from build123d import *

# Parameters (mm, degrees)
F0_W      = 76.2
F0_H      = 63.5
F1_DEPTH  = 50.8
F3_DEPTH  = 50.8
F4_W      = 19.05
F4_H      = 44.45
F5_DEPTH  = 38.1
F6_W      = 19.05
F6_H      = 19.05
F7_DEPTH  = 12.7
F10_DEPTH = 12.7
F11_R     = 3.175
F12_DEPTH = 69.851
F13_DEPTH = 31.75


with BuildPart() as f1:
    # F0 (on Front) → F1 (new body)
    with BuildSketch(Plane.XZ):
        with Locations((-7.4970987678, 21.3185883239)):
            Rectangle(F0_W, F0_H)
    extrude(amount=-F1_DEPTH)

    # F2 (on face) → F3 (cut)
    with BuildSketch(Plane.XZ):
        Polygon((-45.5970987678, 14.9685883239), (-45.5970987678, -10.4314116761), (-20.1970987678, -10.4314116761), align=None)
        Polygon((30.6029012322, 40.3685883239), (30.6029012322, 53.0685883239), (-7.4970987678, 53.0685883239), align=None)
    extrude(amount=-F3_DEPTH, mode=Mode.SUBTRACT)

    # F4 (on face) → F5 (join)
    with BuildSketch(Plane.YZ.offset(30.6029012322)):
        Polygon((19.05, 14.9685883239), (19.05, -10.4314116761), (50.8, -10.4314116761), (50.8, 14.9685883239), (38.1, 14.9685883239), align=None)
        with Locations((28.575, 37.1935883239)):
            Rectangle(F4_W, F4_H)
    extrude(amount=F5_DEPTH)

    # F6 (on face) → F7 (join)
    with BuildSketch(Plane(origin=(30.6029012322, 0, 0), x_dir=(0, -1, 0), z_dir=(-1, 0, 0))):
        with Locations((-28.575, 49.8935883239)):
            Rectangle(F6_W, F6_H)
    extrude(amount=F7_DEPTH)

    # F9 (on face) → F10 (join)
    with BuildSketch(Plane(origin=(0, 38.1, 0), x_dir=(-1, 0, 0), z_dir=(0, 1, 0))):
        Polygon((-30.6029012322, 34.0185883239), (-68.7029012322, 14.9685883239), (-30.6029012322, 14.9685883239), align=None)
    extrude(amount=F10_DEPTH)

    # F11 (on face) → F12 (cut, through all)
    with BuildSketch(Plane.XY.offset(59.4185883239)):
        with Locations((27.4279012322, 28.575)):
            Circle(F11_R)
        with Locations((44.9788695751, 28.575)):
            Circle(F11_R)
    extrude(amount=-F12_DEPTH, mode=Mode.SUBTRACT)

    # F8 (on face) → F13 (cut)
    with BuildSketch(Plane.XZ.offset(-19.05)):
        Polygon((56.0029012322, 59.4185883239), (56.0029012322, 21.3185883239), (68.7029012322, 14.9685883239), (68.7029012322, 59.4185883239), align=None)
    extrude(amount=-F13_DEPTH, mode=Mode.SUBTRACT)


solid = f1.part
Can you work these out from the model? Positions are in its coordinate system, mm. A direction names the side the tool comes from. Give positions to 0.01 mm unless a question says otherwise; leave off trailing zeros. Order: outer loops, then holes, each group sorted by start corner. A loop starts at its lowest first (then second) coordinate and runs counter-clockwise, first axis right, second up. Notation, with made-up numbers: M 44.25,47 L 67.25,47 A14 ccw 67.25,70 Z; hole C 32.25,49 d4. An arc over 180 degrees is marked long. Use a Markdown table: item, result. Add a question column.
Item 1: Suppose I cut it at D-D (z = 38). List the corners of the cut face in (x, y) for me (3 decimals), then the cut area to 3 significant figures.
Item 2: Suppose I cut it at C-C (x = 47). List the corners of the cut face in (y, z) for me, then the cut area to 3 significant figures.
Item 3: Suppose I cut it at A-A (y = 34.5). List the corners of the cut face in (x, z) for me, then the cut area to 3 significant figures.
Item 4: Will these pins go through, and if not, where does the flat tip stop? pin 1 (6 mm diameter, centred on y = 21, z = 19, fed in from +X); pin 2 (15 mm diameter, centred on y = 9, z = 13, fed in from +X); pin 3 (5.5 mm diameter, centred on y = 25.5, z = 43.5, fed in from +X).
Item 5: If I drill on L1, parallel to X at y = 42, z = 35; L2, parallel to Y at x = 41, z = 2.5; L3, parallel to Y at x = 28.5, z = 23.5, over which ranges is the centre line in solid material (lowest first)? Write a range as [from, to].
Item 6: We'd pull the mould along Y, two halves only. Please class faces 1 (the flat face through (12, 50.8, 22)), 2 (the cylindrical face through (42.46, 26.64, 24.98)), 3 (the flat face through (53.62, 41.76, 22.51)): +Y half, -Y half, draft (parallel to the pull), parting line (faces both ways), or undercut.
Item 7: Suppose I cut it at B-B (z = 50). List the corners of the cut face in (x, y) for me (3 decimals).
Item 8: For faces 4 (the flat face through (30.603, 44, 37)), 5 (the flat face through (-27, 25, 53.069)), 6 (the flat face through (56.003, 28, 41)), 7 (the flat face through (30.603, 9, 15)), 8 (the flat face through (17.903, 29, 52)), which set-ups out of +Z, -Z, +X, -X, +Y, -Y let a thin tool reach every point of the face, with its end or its side?
Answer sheet:
| question | item | result |
|---|---|---|
| 1 | outline | M -45.597,0 L 30.603,0 L 30.603,19.05 L 56.003,19.05 L 56.003,38.1 L 30.603,38.1 L 30.603,50.8 L -45.597,50.8 Z; hole C 27.428,28.575 d6.35; hole C 44.979,28.575 d6.35 |
| 1 | area | 4,290 mm² |
| 2 | outline | M 19.05,-10.43 L 26.13,-10.43 L 26.13,59.42 L 19.05,59.42 Z; M 31.02,-10.43 L 50.8,-10.43 L 50.8,25.82 L 38.1,25.82 L 38.1,59.42 L 31.02,59.42 Z |
| 2 | area | 1,450 mm² |
| 3 | outline | M -45.6,14.97 L -20.2,-10.43 L 68.7,-10.43 L 68.7,14.97 L 56,21.32 L 56,59.42 L 17.9,59.42 L 17.9,44.6 L -7.5,53.07 L -45.6,53.07 Z |
| 3 | area | 6,630 mm² |
| 4 | pin 1 | stops at x = 66.64 |
| 4 | pin 2 | stops at x = 30.6 |
| 4 | pin 3 | stops at x = 56 |
| 5 | L1 | x = [-45.6, 30.6] |
| 5 | L2 | y = [19.05, 50.8] |
| 5 | L3 | y = [0, 25.59], [31.56, 50.8] |
| 6 | face 1 | +Y half |
| 6 | face 2 | undercut |
| 6 | face 3 | draft |
| 7 | outline | M -45.597,0 L 1.709,0 L 1.709,50.8 L -45.597,50.8 Z; M 17.903,19.05 L 56.003,19.05 L 56.003,38.1 L 17.903,38.1 Z; hole C 27.428,28.575 d6.35; hole C 44.979,28.575 d6.35 |
| 8 | face 4 | +Z, +X, +Y |
| 8 | face 5 | +Z, -X, +Y, -Y |
| 8 | face 6 | +Z, +X, +Y, -Y |
| 8 | face 7 | +Z, -Z, +X, -Y |
| 8 | face 8 | +Z, +Y, -Y |
